For this review, take the finished solid that the model builds, in its own axes (mm). Face numbers are marked on the shaded views. A direction names the side the tool comes from. Give positions to 0.01 mm unless a question says otherwise; leave off trailing zeros. Order: outer loops, then holes, each group sorted by start corner. A loop starts at its lowest first (then second) coordinate and runs counter-clockwise, first axis right, second up. Notation, with made-up numbers: (53.5, 15) - (87.5, 15) arc R27 ccw to (87.5, 48) - close; hole circle Ø4 at (40, -25.5). An arc over 180 degrees is marked (long way). One line per item, written item: value.
```python
from build123d import *

# Parameters (mm, degrees)
SKETCH1_W   = 9.525
SKETCH1_H   = 6.35
SKETCH1_W_2 = 3.175
SKETCH1_H_2 = 19.05


with BuildPart() as part:
    # Sketch1 → Revolve1 (revolve)
    with BuildSketch(Plane.XY, mode=Mode.PRIVATE) as revolve1_sk:
        with Locations((7.9375, 3.175)):
            Rectangle(SKETCH1_W, SKETCH1_H)
        with Locations((1.5875, 9.525)):
            Rectangle(SKETCH1_W_2, SKETCH1_H_2)
    revolve1 = revolve(revolve1_sk.sketch.rotate(Axis((0, 0, 0), (1, 0, 0)), 90), axis=Axis((0, 0, 0), (1, 0, 0)))

    # Mirror1: Revolve1 across Right Plane
    add(revolve1.mirror(Plane(origin=(0, 0, 0), x_dir=(0, 0, -1), z_dir=(1, 0, 0))))

    # Sketch3 → 1/4-28 Tapped Hole1 (revolve, cut)
    with BuildSketch(Plane(origin=(12.7, 0, 0), x_dir=(0, 0, -1), z_dir=(0, 1, 0))):
        Polygon((0, 0), (0, 25.4), (3.3401, 25.4), (2.7051, 24.765), (2.7051, 1.1049), (3.81, 0), align=None)
    revolve(axis=Axis((19.05, 0, 0), (-1, 0, 0)), mode=Mode.SUBTRACT)


solid = part.part
```
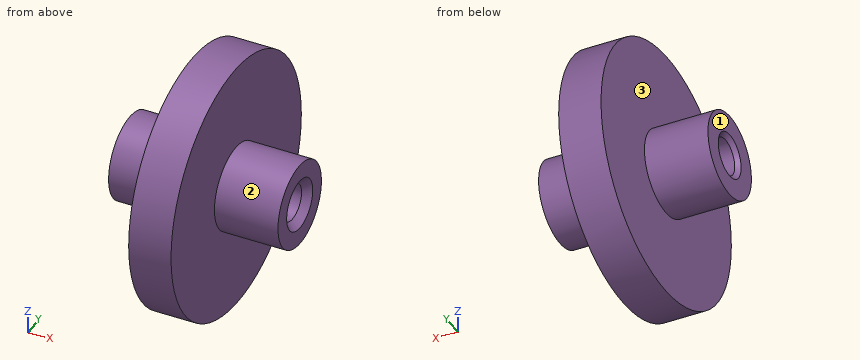
(1) Take a section at C-C (x = -7.5). Write out the cut boundary in (y, z), then the cut area to 3 significant figures.
Answers below:
outline: circle Ø12.7 at (0, 0); hole circle Ø5.41 at (0, 0)
area: 104 mm^2
(2) Wall thickness on line 1 (Y direction, x = 0, z = 0); line 2 (Y direction, x = -4.5, z = 0); line 3 (X direction, y = -10.5, z = 2.5) (3 decimals): over which ranges is each line inside the solid? List them lowest first. Write a range as from..to.
Answers below:
line 1: y = -19.05..-2.71, 2.71..19.05
line 2: y = -6.35..-2.71, 2.71..6.35
line 3: x = -3.175..3.175
(3) Take a section at A-A (y = 0). Write out the cut boundary in (x, z) (3 decimals).
Answers below:
outline: (-12.7, -6.35) - (-3.175, -6.35) - (-3.175, -19.05) - (3.175, -19.05) - (3.175, -6.35) - (12.7, -6.35) - (12.7, -3.81) - (11.595, -2.705) - (-12.065, -2.705) - (-12.7, -3.34) - close; (-12.7, 3.34) - (-12.065, 2.705) - (11.595, 2.705) - (12.7, 3.81) - (12.7, 6.35) - (3.175, 6.35) - (3.175, 19.05) - (-3.175, 19.05) - (-3.175, 6.35) - (-12.7, 6.35) - close
(4) Take a section at D-D (y = -5). Write out the cut boundary in (x, z) (3 decimals), then the cut area to 3 significant figures.
Answers below:
outline: (-12.7, -3.914) - (-3.175, -3.914) - (-3.175, -18.382) - (3.175, -18.382) - (3.175, -3.914) - (12.7, -3.914) - (12.7, 3.914) - (3.175, 3.914) - (3.175, 18.382) - (-3.175, 18.382) - (-3.175, 3.914) - (-12.7, 3.914) - close
area: 383 mm^2
(5) For P1, Ø1, axis at y = 6.5, z = -12, coming from the -X side (3 decimals); P2, Ø6, axis at x = -5.5, y = -9.5, coming from the +Z side; P3, Ø4, axis at x = -1.5, y = 8.5, coming from the -Z side, all flat-tipped, find the tip position at first contact; note any pin that passes through.
Answers below:
P1: stops at x = -3.175
P2: stops at z = 17.47
P3: stops at z = -17.91
(6) Machinability: for the marked faces 1, 2 and 3, which of the approach directions +Z, -Z, +X, -X, +Y, -Y give a long, thin tool a straight path to every point of the face, cutting with its end or side? Answer none if there is none.
Answers below:
face 1: +Z, -Z, -X, +Y, -Y
face 2: +X
face 3: -X
